For this review, use the dimensioned drawing (mm, ordinates from the lowest corner) and the shaded views. Coordinates: 2 decimals unless noted, no trailing zeros. Loops run counter-clockwise (first coordinate to the right, second up) from the corner with the lowest first, then second, coordinate; pieces in that order, holes last. Notation, with made-up numbers: M 6.5,47 L 31.5,47 A16 ccw 31.5,57 Z; hole C 28.25,-18.75 d10. An arc over 180 degrees is marked long. Write item = value, one per line. Start each with the question number.
Q1. Mouldability with a two-part tool opening along Z and no side actions: class the marked faces 1, 2 and 3 as released by +Z, released by -Z, zero draft, split by the parting line, or undercut.
Q2. Clearance check with flat-ended pins moving along their axes: pin 1 Ø4 at (x, z) = (1210.5, 67) entering from -Y; pin 2 Ø8 at (x, y) = (801, 97.5) entering from +Z. State where each tip first meets the part, or that it passes through.
Q3. Wall thickness on probe 1 along Z at (x, y) = (1526.5, 155.5); probe 2 along Y at (x, z) = (539.5, 52.5): over which ranges is each line inside the solid? List them lowest first.
Q4. We need section A-A on z = 72.5. Give the boundary of the cut face in (x, y), and give its area (3 significant figures).
Q5. We need section B-B on x = 768.5. Give the boundary of the cut face in (y, z).
Q6. We need section C-C on y = 99. Give the boundary of the cut face in (x, z), and give its area (3 significant figures).
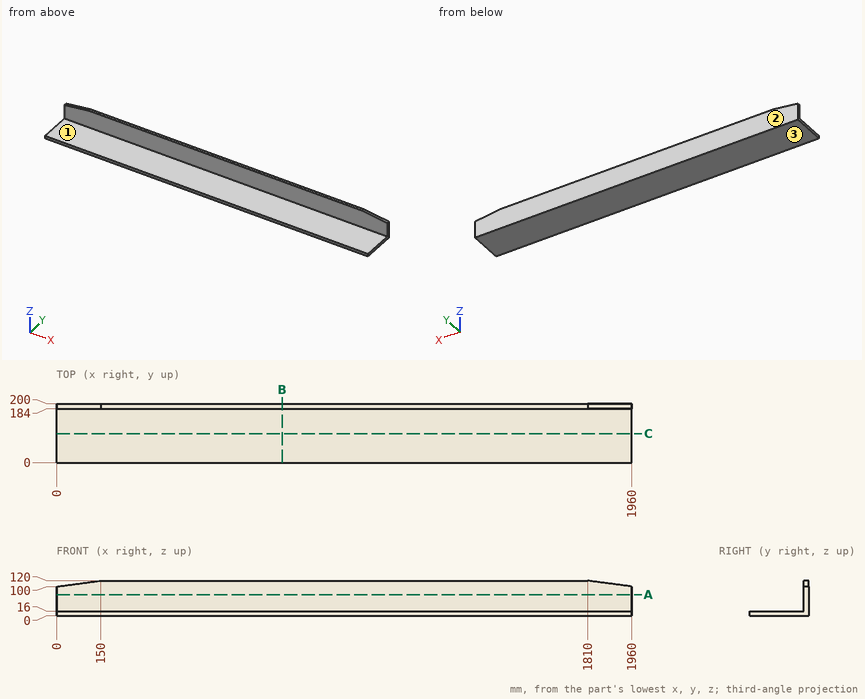
Returned:
q1.face_1 = released by +Z
q1.face_2 = zero draft
q1.face_3 = released by -Z
q2.pin_1 = 184
q2.pin_2 = 16
q3.probe_1 = 0 to 16
q3.probe_2 = 184 to 200
q4.outline = M 0,184 L 1960,184 L 1960,200 L 0,200 Z
q4.area = 31,400 mm^2
q5.outline = M 0,0 L 200,0 L 200,120 L 184,120 L 184,16 L 0,16 Z
q6.outline = M 0,0 L 1960,0 L 1960,16 L 0,16 Z
q6.area = 31,400 mm^2
